```python
from build123d import *

# Parameters (mm, degrees)
SKETCH1_R           = 1.4224
BOSS_EXTRUDE1_DEPTH = 1.5875


with BuildPart() as part:
    # Sketch1 → Boss-Extrude1 (new body)
    with BuildSketch(Plane.XY):
        with BuildLine():
            Line((-14.952058744, -2.948480848), (-16.984058744, -2.948480848))
            Line((-16.984058744, -2.948480848), (-16.984058744, -5.5245))
            Line((-16.984058744, -5.5245), (-20.871224203, -5.5245))
            ThreePointArc((-20.871224203, -5.5245), (21.59, 0), (-20.871224203, 5.5245))
            Line((-20.871224203, 5.5245), (-16.984058744, 5.5245))
            Line((-16.984058744, 5.5245), (-16.984058744, 2.948480848))
            Line((-16.984058744, 2.948480848), (-14.952058744, 2.948480848))
            ThreePointArc((-14.952058744, 2.948480848), (-13.968818521, 6.093415226), (-12.332576282, 8.9535))
            Line((-12.332576282, 8.9535), (-7.9248, 7.366))
            Line((-7.9248, 7.366), (-7.9248, 3.302))
            Line((-7.9248, 3.302), (-5.6007, 3.302))
            Line((-5.6007, 3.302), (-5.6007, 14.173558463))
            ThreePointArc((-5.6007, 14.173558463), (-4.895856129, 14.43219293), (-4.179129857, 14.6558))
            Line((-4.179129857, 14.6558), (4.179129857, 14.6558))
            Line((4.179129857, 14.6558), (11.43, 14.6558))
            Line((11.43, 14.6558), (11.43, -0.8128))
            Line((11.43, -0.8128), (12.9413, -0.8128))
            Line((12.9413, -0.8128), (12.9413, -4.064))
            Line((12.9413, -4.064), (8.4582, -4.064))
            Line((8.4582, -4.064), (8.4582, -8.9154))
            Line((8.4582, -8.9154), (1.2573, -8.9154))
            Line((1.2573, -8.9154), (1.2573, -7.3406))
            Line((1.2573, -7.3406), (-0.7747, -8.8265))
            Line((-0.7747, -8.8265), (-3.273729572, -11.3919))
            Line((-3.273729572, -11.3919), (-5.093162196, -9.619538602))
            Line((-5.093162196, -9.619538602), (-4.769706241, -9.287492148))
            Line((-4.769706241, -9.287492148), (-9.167166743, -5.0038))
            Line((-9.167166743, -5.0038), (-14.395123673, -5.0038))
            ThreePointArc((-14.395123673, -5.0038), (-14.709533071, -3.985879682), (-14.952058744, -2.948480848))
        make_face()
        with Locations((0, 18.415)):
            Circle(SKETCH1_R, mode=Mode.SUBTRACT)
        with Locations((0, -18.415)):
            Circle(SKETCH1_R, mode=Mode.SUBTRACT)
    extrude(amount=BOSS_EXTRUDE1_DEPTH)


solid = part.part
```
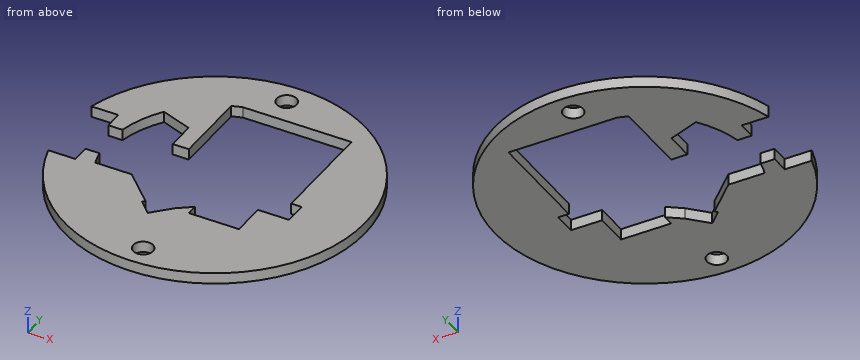
Here's how the part is built. I have some questions about the finished solid (model axes, mm). Coordinates: 2 decimals unless noted, no trailing zeros. Order: outer loops, then holes, each group sorted by start corner. A loop starts at its lowest first (then second) coordinate and runs counter-clockwise, first axis right, second up.
Item 1: If we section it at A-A, the plane x = 2: List the corners of the cut face in (y, z) for me, then the cut area to 3 significant figures.
Response values:
outline: (-21.5, 0) - (-8.92, 0) - (-8.92, 1.59) - (-21.5, 1.59) - close; (14.66, 0) - (21.5, 0) - (21.5, 1.59) - (14.66, 1.59) - close
area: 30.8 mm2
Item 2: If we section it at B-B, the plane y = 13.5: List the corners of the cut face in (x, z) for me.
Response values:
outline: (-16.85, 0) - (-5.6, 0) - (-5.6, 1.59) - (-16.85, 1.59) - close; (11.43, 0) - (16.85, 0) - (16.85, 1.59) - (11.43, 1.59) - close
Item 3: I need wall thicknesses on probe 1 along Y at (x, z) = (0, 0.5); probe 2 along X at (y, z) = (4, 0.1); probe 3 along X at (y, z) = (14, 0.5). Which ranges of each line are inside material? Lowest first, please.
Response values:
probe 1: y = -21.59 to -19.84, -16.99 to -8.26, 14.66 to 16.99, 19.84 to 21.59
probe 2: x = -16.98 to -14.71, -7.92 to -5.6, 11.43 to 21.22
probe 3: x = -16.44 to -5.6, 11.43 to 16.44
Item 4: If we section it at D-D, the plane y = 0: List the corners of the cut face in (x, z) for me, then the cut area to 3 significant figures.
Response values:
outline: (11.43, 0) - (21.59, 0) - (21.59, 1.59) - (11.43, 1.59) - close
area: 16.1 mm2
Item 5: I'm going to push flat-ended pins straight in: pin 1 Ø10 at (x, y) = (2.5, -1) entering from -Z; pin 2 Ø0.8 at (x, z) = (6.5, 0.5) entering from +Y; pin 3 Ø0.5 at (x, z) = (-18.5, 1) entering from +Y; pin 4 Ø0.5 at (x, z) = (6.5, 1) entering from -Y. Where does each tip first touch, or does it pass through?
Response values:
pin 1: passes through
pin 2: stops at y = 20.71
pin 3: stops at y = 11.54
pin 4: stops at y = -20.67
Item 6: If we section it at C-C, the plane z = 1.25: Give the number of separate pieces and of enclosed holes in the cut face, then the cut area to 3 significant figures.
Response values:
separate pieces: 1
enclosed holes: 2
area: 883 mm2
